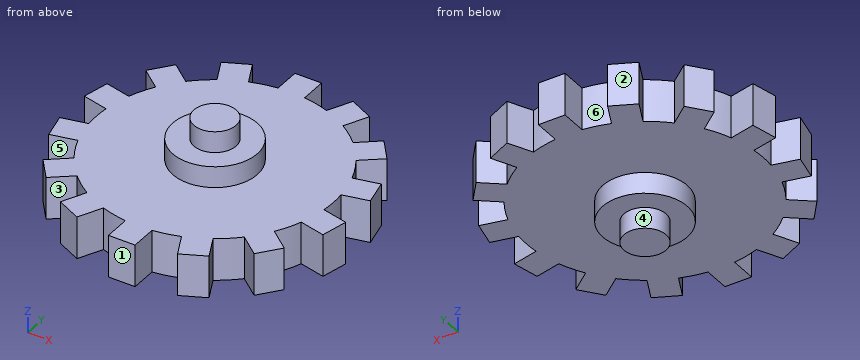
from build123d import *

# Parameters (mm, degrees)
SKETCH2_R           = 28
BOSS_EXTRUDE1_DEPTH = 5
SKETCH5_W           = 6.3
SKETCH5_H           = 12
BOSS_EXTRUDE2_DEPTH = 10
CIRPATTERN1_COUNT   = 14
SKETCH6_R           = 10
BOSS_EXTRUDE3_DEPTH = 5
SKETCH7_R           = 5
BOSS_EXTRUDE4_DEPTH = 5


with BuildPart() as part:
    # Sketch2 → Boss-Extrude1 (new, symmetric)
    with BuildSketch(Plane.XY):
        Circle(SKETCH2_R)
    extrude(amount=BOSS_EXTRUDE1_DEPTH, both=True)

    # Sketch5 → Boss-Extrude2 (add)
    with BuildSketch(Plane.XY.offset(5)):
        with Locations((0, 28)):
            Rectangle(SKETCH5_W, SKETCH5_H)
    boss_extrude2 = extrude(amount=-BOSS_EXTRUDE2_DEPTH)

    # CirPattern1: Boss-Extrude2 ×14 about axis
    cirpattern1_axis = Axis((0, 0, 0), (0, 0, 1))
    for i in range(1, CIRPATTERN1_COUNT):
        add(boss_extrude2.rotate(cirpattern1_axis, i * 360 / CIRPATTERN1_COUNT))

    # Sketch6 → Boss-Extrude3 (add)
    with BuildSketch(Plane.XY.offset(5)):
        Circle(SKETCH6_R)
    boss_extrude3 = extrude(amount=BOSS_EXTRUDE3_DEPTH)

    # Sketch7 → Boss-Extrude4 (add)
    with BuildSketch(Plane.XY.offset(10)):
        Circle(SKETCH7_R)
    boss_extrude4 = extrude(amount=BOSS_EXTRUDE4_DEPTH)

    # Mirror1: Boss-Extrude3, Boss-Extrude4 across plane
    add(boss_extrude3.mirror(Plane.XY))
    add(boss_extrude4.mirror(Plane.XY))


solid = part.part
Build history of the part. All positions in model axes, mm. Face numbers are marked on the shaded views. A direction names the side the tool comes from. Round coordinates to 2 decimals unless told otherwise and drop trailing zeros. Write each loop counter-clockwise with the first axis right and the second up, starting at its lowest first coordinate (ties: lowest second). Pieces come first, ordered by that corner, then holes. Notation, with made-up numbers: M 68,16 L 82,16 A11 cw 82,25 Z; hole C -23,5 d9. An arc over 180 degrees is marked long. Answer as a JSON object with one key per item and string values. Group by question number.
(1) Cut at A-A (x = -16). Give the cut face in (y, z), and give its area (3 significant figures).
(2) Cut at D-D (y = 0). Give the cut face in (x, z).
(3) Drill centre lines: L1, parallel to Y at x = 27, z = 3.75; L2, parallel to Z at x = 3, y = 16; L3, parallel to Y at x = -16, z = -3.5. Where is each one in solid material? Low to high.
(4) Flat gauge pins, fed straight in: pin 1 (8 mm diameter, centred on y = 12, z = 3, fed in from -X); pin 2 (5 mm diameter, centred on x = 22.5, y = 5.5, fed in from +Z); pin 3 (3 mm diameter, centred on x = -19, z = 2, fed in from +Y). Where does each tip first touch, or does it go through?
(5) Which spindle directions (+Z, -Z, +X, -X, +Y, -Y) get a long thin tool onto all of the face, cutting with end or side? Do the marked faces 4, 5 and 6. Say none if no direction does.
(6) Cut at C-C (x = 0). Give the cut face in (y, z).
(7) Mould opens along X. For the marked faces 1, 2 and 3 say: pulls with the +X half, pulls with the -X half, needs draft (parallel to the pull), parting line crosses it, or undercut.
(8) Cut at B-B (y = 21.5). Give the cut face in (x, z).
Responses:
{
 "1": {"outline": "M -30.03,-5 L -25.96,-5 L -25.96,5 L -30.03,5 Z; M -22.98,-5 L 22.98,-5 L 22.98,5 L -22.98,5 Z; M 25.96,-5 L 30.03,-5 L 30.03,5 L 25.96,5 Z", "area": "541 mm2"},
 "2": {"outline": "M -28,-5 L -10,-5 L -10,-10 L -5,-10 L -5,-15 L 5,-15 L 5,-10 L 10,-10 L 10,-5 L 28,-5 L 28,5 L 10,5 L 10,10 L 5,10 L 5,15 L -5,15 L -5,10 L -10,10 L -10,5 L -28,5 Z"},
 "3": {"L1": "y = -20.67 to -17.5, -9.39 to 9.39, 17.5 to 20.67", "L2": "z = -5 to 5", "L3": "y = -30.03 to -25.96, -22.98 to 22.98, 25.96 to 30.03"},
 "4": {"pin 1": "stops at x = -33.05", "pin 2": "stops at z = 5", "pin 3": "stops at y = 29.31"},
 "5": {"face 4": "-Z", "face 5": "+Z, -Z", "face 6": "+Z, -Z, +Y"},
 "6": {"outline": "M -34,-5 L -10,-5 L -10,-10 L -5,-10 L -5,-15 L 5,-15 L 5,-10 L 10,-10 L 10,-5 L 34,-5 L 34,5 L 10,5 L 10,10 L 5,10 L 5,15 L -5,15 L -5,10 L -10,10 L -10,5 L -34,5 Z"},
 "7": {"face 1": "needs draft", "face 2": "pulls with the -X half", "face 3": "undercut"},
 "8": {"outline": "M -26.34,-5 L -21.91,-5 L -21.91,5 L -26.34,5 Z; M -17.94,-5 L 17.94,-5 L 17.94,5 L -17.94,5 Z; M 21.91,-5 L 26.34,-5 L 26.34,5 L 21.91,5 Z"}
}
